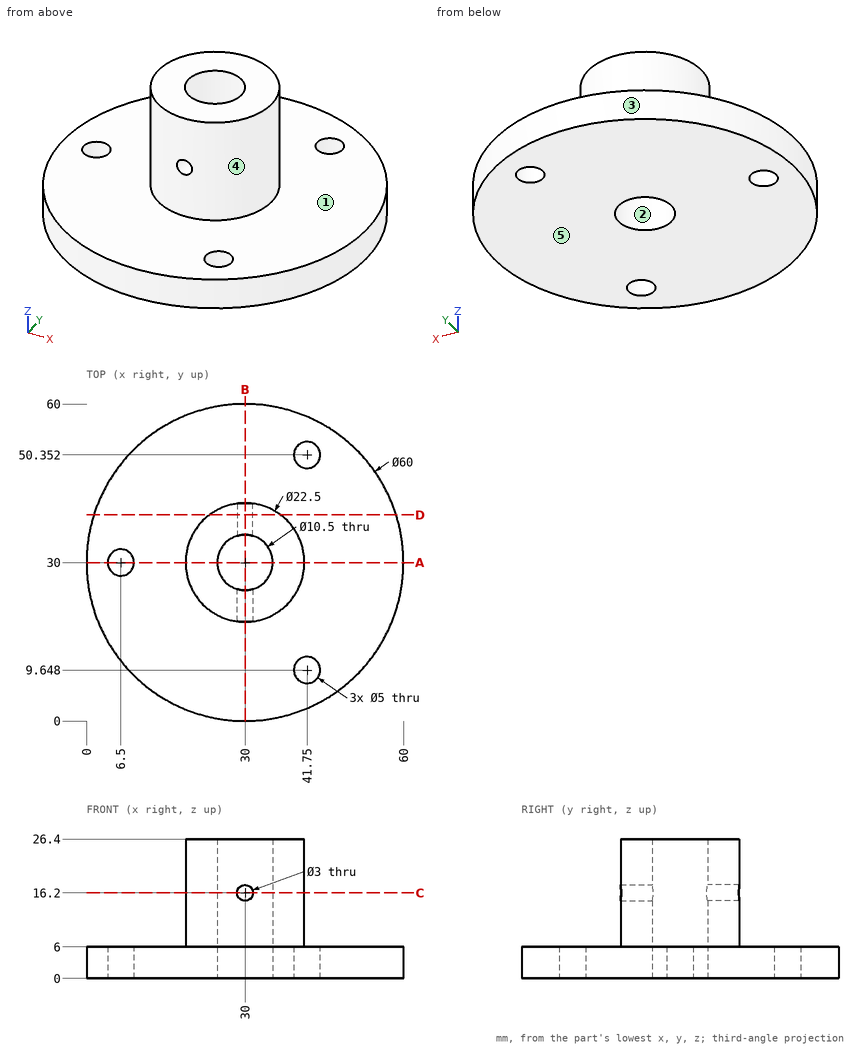
Check sheet for the drawn part. Datum: minimum x, y, z corner. Units: mm. A direction names the side the tool comes from. Coordinates: 2 decimals unless noted, no trailing zeros. Order: outer loops, then holes, each group sorted by start corner. A loop starts at its lowest first (then second) coordinate and runs counter-clockwise, first axis right, second up. Notation, with made-up numbers: M -6,-17.75 L 52,-17.75 A11 cw 52,-12.75 Z; hole C 35.5,2 d5. An arc over 180 degrees is marked long. One line per question, with ' | ' between items. Start each with the question number.
Item 1: Sectioned sample at B-B on x = 30. Record the cut outline in (y, z), and give its area (3 significant figures).
Item 2: Sectioned sample at A-A on y = 30. Record the cut outline in (x, z), and give its area (3 significant figures).
Item 3: Mould release check, pull along Y, two halves, no side actions. Record for the marked faces 1, 2 and 3: pulls with the +Y half, pulls with the -Y half, needs draft (parallel to the pull), parting line crosses it, or undercut.
Item 4: Gauge pin test, flat ends, axial feed: P1, Ø10, axis at y = 34.5, z = 16.5, coming from the -X side; P2, Ø2, axis at y = 29.5, z = 23, coming from the +X side; P3, Ø8, axis at x = 41.75, y = 9.65, coming from the -Z side; P4, Ø8, axis at x = 46.5, z = 16, coming from the -Y side. Record the tip position at first contact, or that the pin passes through.
Item 5: Sectioned sample at D-D on y = 39. Record the cut outline in (x, z).
Item 6: Access from +Z, -Z, +X, -X, +Y, -Y to the whole of each face (thin tool, end or side, straight path). Record for the marked faces 4 and 5.
Item 7: Sectioned sample at C-C on z = 16.2. Record the cut outline in (x, y), and give its area (3 significant figures).
Item 8: Material ranges on line 1 (Z direction, x = 8, y = 17); line 2 (Y direction, x = 30, z = 13.25); line 3 (Y direction, x = 41.75, z = 3.15), recorded low to high.
Answer below:
1) outline: M 0,0 L 24.75,0 L 24.75,14.7 L 18.75,14.7 L 18.75,6 L 0,6 Z; M 18.75,17.7 L 24.75,17.7 L 24.75,26.4 L 18.75,26.4 Z; M 35.25,0 L 60,0 L 60,6 L 41.25,6 L 41.25,14.7 L 35.25,14.7 Z; M 35.25,17.7 L 41.25,17.7 L 41.25,26.4 L 35.25,26.4 Z | area: 506 mm^2
2) outline: M 0,0 L 4,0 L 4,6 L 0,6 Z; M 9,0 L 24.75,0 L 24.75,26.4 L 18.75,26.4 L 18.75,6 L 9,6 Z; M 35.25,0 L 60,0 L 60,6 L 41.25,6 L 41.25,26.4 L 35.25,26.4 Z | area: 512 mm^2
3) face 1: needs draft | face 2: undercut | face 3: parting line crosses it
4) P1: stops at x = 18.75 | P2: stops at x = 41.25 | P3: stops at z = 0 | P4: passes through
5) outline: M 1.38,0 L 58.62,0 L 58.62,6 L 36.75,6 L 36.75,26.4 L 23.25,26.4 L 23.25,6 L 1.38,6 Z; hole C 30,16.2 d3
6) face 4: +Z | face 5: -Z, +X, -X, +Y, -Y
7) outline: M 28.5,18.85 L 28.5,24.97 A5.25 cw 28.5,35.03 L 28.5,41.15 A11.25 ccw Z; M 31.5,18.85 A11.25 ccw 31.5,41.15 L 31.5,35.03 A5.25 cw 31.5,24.97 Z | area: 275 mm^2
8) line 1: z = 0 to 6 | line 2: y = 18.75 to 24.75, 35.25 to 41.25 | line 3: y = 2.4 to 7.15, 12.15 to 47.85, 52.85 to 57.6
